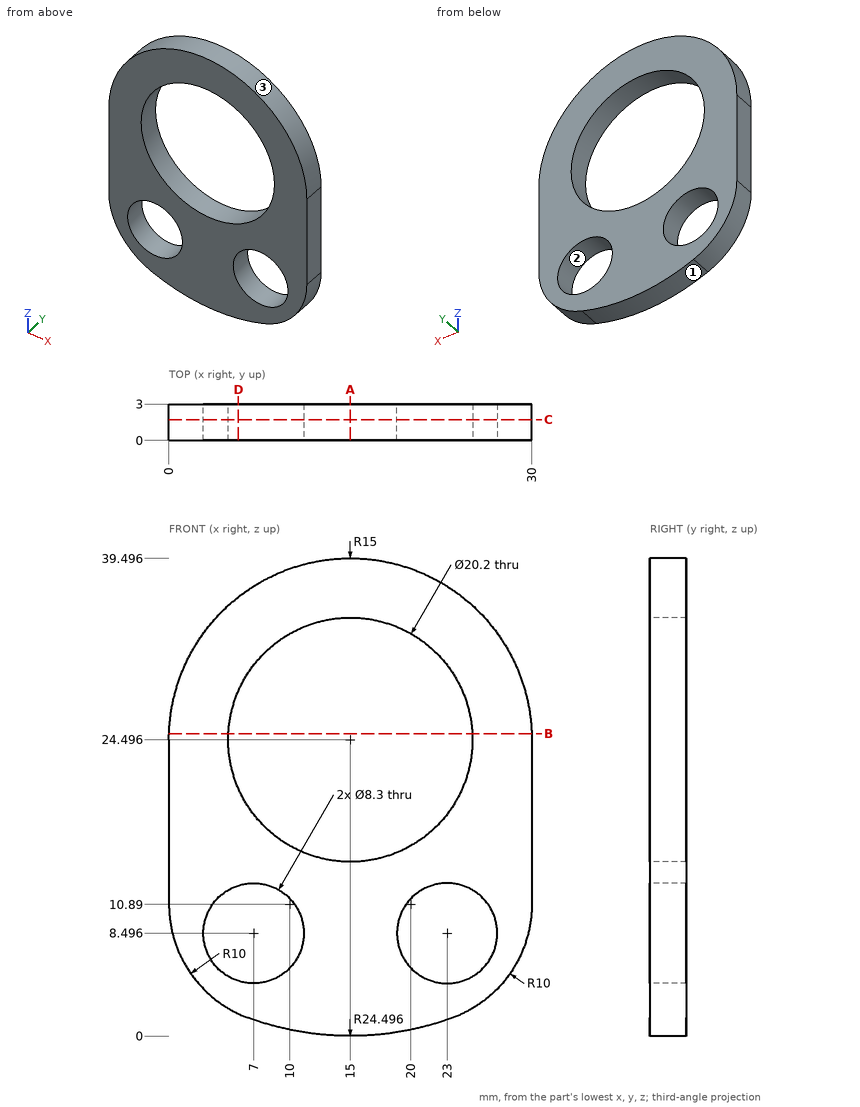
Verification items for this drawing (mm, ordinates from the low corner). Coordinates: 2 decimals unless noted, no trailing zeros. Write each loop counter-clockwise with the first axis right and the second up, starting at its lowest first coordinate (ties: lowest second). Pieces come first, ordered by that corner, then holes. Notation, with made-up numbers: (-24.5, -27) -> (34.5, -27) arc R29 ccw to (34.5, -6) -> close; hole circle Ø2 at (-24, 47.25). An arc over 180 degrees is marked (long way). One line per item, written item: value. Start each with the question number.
Q1. Go/stop test with a flat-tipped pin: P1, Ø1, axis at y = 0.5, z = 27.5, coming from the +X side. Record where the tip stops, or that it passes through.
Q2. Cross-section at D-D on x = 5.75. Enter the section's corners in (y, z).
Q3. Thickness scan on L1, parallel to X at y = 1.6, z = 8.5; L2, parallel to Z at x = 7, y = 2.05 (1 decimal); L3, parallel to Z at x = 15, y = 1.15 (1 decimal). Record the ranges inside material, lowest first. Write a range as from..to.
Q4. Cross-section at C-C on y = 1.7. State how many separate pieces and enclosed holes the cut face has, and give its area (3 significant figures).
Q5. Cross-section at B-B on z = 25. Enter the section's corners in (x, y), and give its area (3 significant figures).
Q6. Mould release check, pull along Z, two halves, no side actions. Record for the marked faces 1, 2 and 3: pulls with the +Z half, pulls with the -Z half, needs draft (parallel to the pull), parting line crosses it, or undercut.
Q7. Cross-section at A-A on x = 15. Enter the section's corners in (y, z) (1 decimal).
Checked values:
1. P1: stops at x = 29.79
2. outline: (0, 1.84) -> (3, 1.84) -> (3, 4.54) -> (0, 4.54) -> close; (0, 12.45) -> (3, 12.45) -> (3, 20.44) -> (0, 20.44) -> close; (0, 28.55) -> (3, 28.55) -> (3, 36.3) -> (0, 36.3) -> close
3. L1: x = 0.29..2.85, 11.15..18.85, 27.15..29.71
3. L2: z = 1.3..4.3, 12.6..18.3, 30.7..37.2
3. L3: z = 0..14.4, 34.6..39.5
4. separate pieces: 1
4. enclosed holes: 3
4. area: 598 mm²
5. outline: (0.01, 0) -> (4.91, 0) -> (4.91, 3) -> (0.01, 3) -> close; (25.09, 0) -> (29.99, 0) -> (29.99, 3) -> (25.09, 3) -> close
5. area: 29.4 mm²
6. face 1: pulls with the -Z half
6. face 2: undercut
6. face 3: pulls with the +Z half
7. outline: (0, 0) -> (3, 0) -> (3, 14.4) -> (0, 14.4) -> close; (0, 34.6) -> (3, 34.6) -> (3, 39.5) -> (0, 39.5) -> close
